Verification items for the finished model (mm, model axes). A direction names the side the tool comes from. Coordinates: 2 decimals unless noted, no trailing zeros. Order: outer loops, then holes, each group sorted by start corner. A loop starts at its lowest first (then second) coordinate and runs counter-clockwise, first axis right, second up. Notation, with made-up numbers: (78, 9.5) -> (111, 9.5) arc R22 cw to (111, 42.5) -> close; hole circle Ø11 at (-4.75, 72.5). An arc over 180 degrees is marked (long way). Use CSV: the item, a comma, the result in double quotes. Start each with the question number.
1) Go/stop test with flat-tipped pins: pin 1 (1 mm diameter, centred on y = 34.5, z = -12.5, fed in from +X); pin 2 (10 mm diameter, centred on y = 27.5, z = -0.5, fed in from -X); pin 3 (4 mm diameter, centred on y = 51, z = 15.5, fed in from +X). Record where each tip stops, or that it passes through.
2) Sectioned sample at A-A on y = 8. Record the boundary of the cut face in (x, z).
3) Sectioned sample at D-D on y = 54. Record the boundary of the cut face in (x, z), then the cut area to 3 significant figures.
4) Sectioned sample at C-C on z = 5. Give the number of separate pieces and of enclosed holes in the cut face, then the cut area to 3 significant figures.
5) Tool access check on faces 5 (the cylindrical face through (17.084, 7.535, 3.794)), 6 (the flat face through (0, 37.5, -16)), 7 (the cylindrical face through (19, 30, 0)), 8 (the flat face through (14, 32, 0)). Record the directions out of +Z, -Z, +X, -X, +Y, -Y that give a thin tool (end or side, any length) a straight path to the whole face; none if there is none.
6) Sectioned sample at B-B on y = 32.5. Record the boundary of the cut face in (x, z), then the cut area to 3 significant figures.
7) Release check for a two-part mould opening along Z. For faces 1 (the flat face through (0, 57, 0)), 2 (the cylindrical face through (-0.769, 27.675, 17.483)), 3 (the cylindrical face through (-6.11, 58.52, 3.99)), 4 (the flat face through (-8, 0, 13)) record: released by +Z, released by -Z, zero draft, split by the parting line, or undercut.
8) Scan lines: line 1 along X through (y, z) = (58, 5); line 2 along Z through (x, y) = (-0.5, 38.5); line 3 along X through (y, z) = (57.5, -6). Record each from-to range of solid material in increasing order.
from build123d import *

# Parameters (mm, degrees)
SKETCH2_R           = 2.5
BOSS_EXTRUDE1_DEPTH = 7.5
SKETCH4_R           = 20
SKETCH4_R_2         = 17.5
BOSS_EXTRUDE3_DEPTH = 2.5
BOSS_EXTRUDE4_START = 2.5
SKETCH5_R           = 20
SKETCH5_R_2         = 17.5
BOSS_EXTRUDE4_DEPTH = 2.5
SKETCH6_R           = 1.5
CUT_EXTRUDE1_DEPTH  = 67.800074972
CIRPATTERN1_COUNT   = 4
SKETCH7_W           = 20
SKETCH7_H           = 10
CUT_EXTRUDE2_DEPTH  = 67.800074882
CHAMFER1_SIZE       = 2.5


with BuildPart() as part:
    # Sketch1 → Revolve1 (revolve)
    with BuildSketch(Plane.XY, mode=Mode.PRIVATE) as revolve1_sk:
        Polygon((15, 0), (17.5, 0), (17.5, 40), (15, 60), (0, 60), (0, 57), (12.875, 57), (15, 40), align=None)
    revolve(revolve1_sk.sketch.rotate(Axis((0, 0, 0), (0, 1, 0)), 90), axis=Axis((0, 0, 0), (0, 1, 0)))

    # Sketch2 → Boss-Extrude1 (add)
    with BuildSketch(Plane(origin=(14, 0, 0), x_dir=(0, 0, -1), z_dir=(1, 0, 0))):
        with Locations(Location((0, 32.5, 0), (0, 0, 180))):
            Circle(SKETCH2_R)
    extrude(amount=BOSS_EXTRUDE1_DEPTH)

    # Sketch4 → Boss-Extrude3 (add)
    with BuildSketch(Plane(origin=(0, 5, 0), x_dir=(1, 0, 0), z_dir=(0, 1, 0))):
        with Locations(Location((0, 0, 0), (0, 0, 270))):
            Circle(SKETCH4_R)
        with Locations(Location((0, 0, 0), (0, 0, 90))):
            Circle(SKETCH4_R_2, mode=Mode.SUBTRACT)
    extrude(amount=-BOSS_EXTRUDE3_DEPTH)

    # Sketch5 → Boss-Extrude4 (add)
    with BuildSketch(Plane(origin=(0, 10, 0), x_dir=(1, 0, 0), z_dir=(0, 1, 0)).offset(BOSS_EXTRUDE4_START)):
        with Locations(Location((0, 0, 0), (0, 0, 270))):
            Circle(SKETCH5_R)
        with Locations(Location((0, 0, 0), (0, 0, 270))):
            Circle(SKETCH5_R_2, mode=Mode.SUBTRACT)
    extrude(amount=-BOSS_EXTRUDE4_DEPTH)

    # Sketch6 → Cut-Extrude1 (cut, through all)
    with BuildSketch(Plane(origin=(0, 60, 0), x_dir=(1, 0, 0), z_dir=(0, 1, 0))):
        with Locations(Location((-5, 5, 0), (0, 0, 270))):
            Circle(SKETCH6_R)
    cut_extrude1 = extrude(amount=-CUT_EXTRUDE1_DEPTH, mode=Mode.SUBTRACT)

    # CirPattern1: Cut-Extrude1 ×4 about axis
    cirpattern1_axis = Axis((0, 0, 0), (0, 1, 0))
    for i in range(1, CIRPATTERN1_COUNT):
        add(cut_extrude1.rotate(cirpattern1_axis, i * 360 / CIRPATTERN1_COUNT), mode=Mode.SUBTRACT)

    # Sketch7 → Cut-Extrude2 (cut, through all)
    with BuildSketch(Plane.XY):
        with Locations((0, 32.5)):
            Rectangle(SKETCH7_W, SKETCH7_H)
    extrude(amount=-CUT_EXTRUDE2_DEPTH, mode=Mode.SUBTRACT)

    # Chamfer1
    chamfer1_edges = [part.edges().sort_by_distance(p)[0] for p in [
        (0, 2.5, 17.5),
        (0, 12.5, 17.5),
    ]]
    chamfer(chamfer1_edges, length=CHAMFER1_SIZE - 0.0001)  # a hair under: the kernel refuses the full size


solid = part.part
Answers follow:
1,pin 1,"stops at x = 12.74"
1,pin 2,"stops at x = -17.5"
1,pin 3,"stops at x = 8.85"
2,outline,"circle Ø35 at (0, 0); hole circle Ø30 at (0, 0)"
3,outline,"circle Ø31.5 at (0, 0); hole circle Ø26.5 at (0, 0)"
3,area,"228 mm²"
4,separate pieces,"3"
4,enclosed holes,"0"
4,area,"407 mm²"
5,face 5,"none"
5,face 6,"-Z"
5,face 7,"+X"
5,face 8,"-Y"
6,outline,"(-10, -14.36) -> (-10, -11.18) arc R15 cw (long way) to (14.79, 2.5) -> (14, 2.5) -> (14, -2.5) -> (14.79, -2.5) arc R15 cw to (10, -11.18) -> (10, -14.36) arc R17.5 ccw to (17.32, -2.5) -> (21.5, -2.5) -> (21.5, 2.5) -> (17.32, 2.5) arc R17.5 ccw (long way) to start"
6,area,"226 mm²"
7,face 1,"undercut"
7,face 2,"split by the parting line"
7,face 3,"undercut"
7,face 4,"zero draft"
8,line 1,"x = -14.41 to -6.5, -3.5 to 3.5, 6.5 to 14.41"
8,line 2,"z = -17.49 to -14.99, 14.99 to 17.49"
8,line 3,"x = -14.09 to -6.12, -3.88 to 3.88, 6.12 to 14.09"
